Check sheet for the modelled part. Datum: model origin and axes. Units: mm. Round coordinates to 2 decimals unless told otherwise and drop trailing zeros. Loops run counter-clockwise (first coordinate to the right, second up) from the corner with the lowest first, then second, coordinate; pieces in that order, holes last. Notation, with made-up numbers: (20.25, 68.5) -> (54.25, 68.5) arc R16 ccw to (54.25, 79.5) -> close; hole circle Ø7 at (76, 70). An arc over 180 degrees is marked (long way). Use one line per item in the form item = value. Start each with the question number.
(1) Material ranges on probe 1 along Y at (x, z) = (0.25, 11); probe 2 along Z at (x, y) = (4.75, 1.75); probe 3 along Z at (x, y) = (0.5, -2.75), recorded low to high. Write a range as [from, to].
(2) Draft check along Z on faces 1 (the flat face through (0, 0, -5)), 2 (the cylindrical face through (-1.08, -4.88, 19.72)), 3 (the flat face through (0, 0, 45)). Enter one of: released by +Z, released by -Z, zero draft, split by the parting line, or undercut.
(3) Go/stop test with flat-tipped pins: pin 1 (5 mm diameter, centred on x = 5, y = -3.5, fed in from -Z); pin 2 (3 mm diameter, centred on x = 4, z = 20.5, fed in from -Y); pin 3 (4 mm diameter, centred on x = 3, z = 15, fed in from +Y). Record where each tip stops, or that it passes through.
(4) Sectioned sample at A-A (z = 39). Record the cut outline in (x, y), and give its area (3 significant figures).
from build123d import *

# Parameters (mm, degrees)
IZIM1_R                     = 5
Y_KSEKLIK_EKSTR_ZYON1_DEPTH = 40
IZIM2_R                     = 7.5
Y_KSEKLIK_EKSTR_ZYON2_DEPTH = 5
RADYUS1_R                   = 5
Y_KSEKLIK_EKSTR_ZYON3_START = 5
IZIM3_R                     = 7.5
Y_KSEKLIK_EKSTR_ZYON3_DEPTH = 5
RADYUS2_R                   = 5


with BuildPart() as part:
    # Çizim1 → Yükseklik-Ekstrüzyon1 (new body)
    with BuildSketch(Plane.XY):
        Circle(IZIM1_R)
    extrude(amount=Y_KSEKLIK_EKSTR_ZYON1_DEPTH)

    # Çizim2 → Yükseklik-Ekstrüzyon2 (add)
    with BuildSketch(Plane.XY.offset(40)):
        Circle(IZIM2_R)
    extrude(amount=Y_KSEKLIK_EKSTR_ZYON2_DEPTH)

    # Radyus1
    radyus1_edges = [part.edges().sort_by_distance(p)[0] for p in [
        (-7.5, 0, 45),
    ]]
    fillet(radyus1_edges, radius=RADYUS1_R - 0.0001)  # a hair under: the kernel refuses the full size

    # Çizim3 → Yükseklik-Ekstrüzyon3 (add)
    with BuildSketch(Plane(origin=(0, 0, 0), x_dir=(-1, 0, 0), z_dir=(0, 0, -1)).offset(Y_KSEKLIK_EKSTR_ZYON3_START)):
        Circle(IZIM3_R)
    extrude(amount=-Y_KSEKLIK_EKSTR_ZYON3_DEPTH)

    # Radyus2
    radyus2_edges = [part.edges().sort_by_distance(p)[0] for p in [
        (7.5, 0, -5),
    ]]
    fillet(radyus2_edges, radius=RADYUS2_R - 0.0001)  # a hair under: the kernel refuses the full size


solid = part.part
Checks:
q1.probe_1 = [-4.99, 4.99]
q1.probe_2 = [-4.29, 0], [40, 44.29]
q1.probe_3 = [-4.99, 44.99]
q2.face_1 = released by -Z
q2.face_2 = undercut
q2.face_3 = released by +Z
q3.pin_1 = -4.88
q3.pin_2 = -4.33
q3.pin_3 = 4.9
q4.outline = circle Ø10 at (0, 0)
q4.area = 78.5 mm2
